```python
from build123d import *

# Parameters (mm, degrees)
SKETCH1_R           = 11.5
SKETCH1_R_2         = 1.75
BOSS_EXTRUDE1_DEPTH = 2
CUT_EXTRUDE1_DEPTH  = 2
CHAMFER1_SIZE       = 4
CHAMFER1_SIZE2      = 1.865230633
CHAMFER2_SIZE       = 4
CHAMFER2_SIZE2      = 1.865230633


with BuildPart() as part:
    # Sketch1 → Boss-Extrude1 (new body)
    with BuildSketch(Plane(origin=(0, 0, 0), x_dir=(1, 0, 0), z_dir=(0, 1, 0))):
        with Locations(Location((0, 0, 0), (0, 0, 270))):
            Circle(SKETCH1_R)
        with Locations(Location((0, 0, 0), (0, 0, 270))):
            Circle(SKETCH1_R_2, mode=Mode.SUBTRACT)
    extrude(amount=BOSS_EXTRUDE1_DEPTH)

    # Sketch2 → Cut-Extrude1 (cut)
    with BuildSketch(Plane(origin=(0, 2, 0), x_dir=(1, 0, 0), z_dir=(0, 1, 0))):
        with BuildLine():
            Line((-1.45362124, 4.5746022), (-2.346992627, 7.386076469))
            ThreePointArc((-2.346992627, 7.386076469), (-4.178678051, 6.526955626), (-5.725593472, 5.223033543))
            Line((-5.725593472, 5.223033543), (-3.546174021, 3.234911098))
            ThreePointArc((-3.546174021, 3.234911098), (-2.58808447, 4.042501549), (-1.45362124, 4.5746022))
        make_face()
        with BuildLine():
            Line((5.725593472, -5.223033543), (3.546174021, -3.234911098))
            ThreePointArc((3.546174021, -3.234911098), (2.58808447, -4.042501549), (1.45362124, -4.5746022))
            Line((1.45362124, -4.5746022), (2.346992627, -7.386076469))
            ThreePointArc((2.346992627, -7.386076469), (4.178678051, -6.526955626), (5.725593472, -5.223033543))
        make_face()
    extrude(amount=-CUT_EXTRUDE1_DEPTH, mode=Mode.SUBTRACT)

    # Chamfer1
    chamfer1_edges = [part.edges().sort_by_distance(p)[0] for p in [
        (-1.900306933, 2, -5.980339335),
    ]]
    chamfer1_side = [part.faces().sort_by_distance(p)[0] for p in [
        (0, 2, -11.174730881),
    ]]
    chamfer(chamfer1_edges, length=CHAMFER1_SIZE, length2=CHAMFER1_SIZE2, reference=chamfer1_side[0])

    # Chamfer2
    chamfer2_edges = [part.edges().sort_by_distance(p)[0] for p in [
        (1.900306933, 2, 5.980339335),
    ]]
    chamfer2_side = [part.faces().sort_by_distance(p)[0] for p in [
        (-0.343824977, 2, -4.461502083),
    ]]
    chamfer(chamfer2_edges, length=CHAMFER2_SIZE, length2=CHAMFER2_SIZE2, reference=chamfer2_side[0])


solid = part.part
```
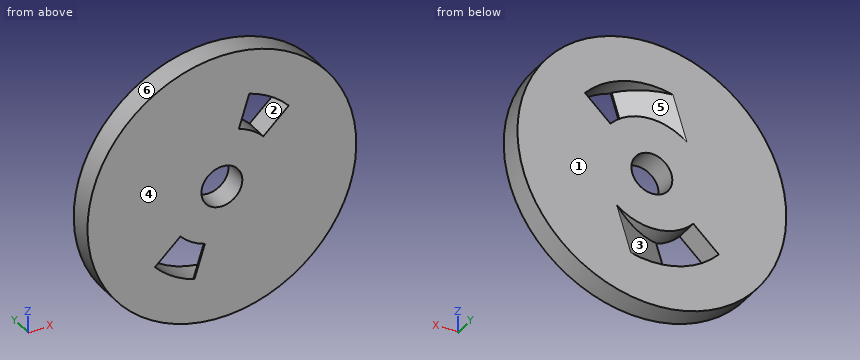
Can you work these out from the model? Positions are in its coordinate system, mm. Face numbers are marked on the shaded views. A direction names the side the tool comes from. Coordinates: 2 decimals unless noted, no trailing zeros. Loops run counter-clockwise (first coordinate to the right, second up) from the corner with the lowest first, then second, coordinate; pieces in that order, holes last. Notation, with made-up numbers: (25, 81.25) -> (81, 81.25) arc R33 ccw to (81, 110.25) -> close; hole circle Ø5 at (16.25, 71.5). An arc over 180 degrees is marked (long way). Answer as a JSON object with one key per item and string values.
1) If I drill on line 1 (Z direction, x = -3.75, y = 1.1); line 2 (X direction, y = 1.1, z = 3.5); line 3 (X direction, y = 0.5, z = 0), over which ranges is the centre line in solid material (lowest first)?
Results:
{"line 1": "z = -10.87 to -6.78, -3.42 to 10.87", "line 2": "x = -10.95 to 3.28, 3.84 to 10.95", "line 3": "x = -11.5 to -1.75, 1.75 to 11.5"}
2) For P1, Ø3, axis at x = 0, z = 0, coming from the -Y side, with a flat end and sliding along its axis, tell me the tip position at first contact or that it passes through.
Results:
{"P1": "passes through"}
3) Imagine slicing it at D-D (x = -5). Please give me the cut outline in (y, z), then the cut area to 3 significant figures.
Results:
{"outline": "(0, -10.36) -> (2, -10.36) -> (2, -5.92) -> (0, -5.92) -> close; (0, -4.56) -> (2, -4.56) -> (2, 10.36) -> (0, 10.36) -> close", "area": "38.7 mm^2"}
4) Imagine slicing it at B-B (x = 0). Please give me the cut outline in (y, z).
Results:
{"outline": "(0, -11.5) -> (2, -11.5) -> (2, -7.75) -> (1.23, -7.75) -> (0.81, -4.8) -> (2, -4.8) -> (2, -1.75) -> (0, -1.75) -> close; (0, 1.75) -> (2, 1.75) -> (2, 4.8) -> (0.81, 4.8) -> (1.23, 7.75) -> (2, 7.75) -> (2, 11.5) -> (0, 11.5) -> close"}
5) Imagine slicing it at C-C (y = 0.55). Please give me the cut outline in (x, z).
Results:
{"outline": "circle Ø23 at (0, 0); hole (-5.73, -5.22) arc R7.75 ccw to (-1.48, -7.61) -> (-0.58, -4.76) arc R4.8 cw to (-3.55, -3.23) -> close; hole circle Ø3.5 at (0, 0); hole (0.58, 4.76) arc R4.8 cw to (3.55, 3.23) -> (5.73, 5.22) arc R7.75 ccw to (1.48, 7.61) -> close"}
6) Thinking about a two-plate mould opening in Z: for the marked faces 4, 5 and 6, which applies, pulls with the +Z half, pulls with the -Z half, needs draft (parallel to the pull), parting line crosses it, or undercut?
Results:
{"face 4": "needs draft", "face 5": "undercut", "face 6": "parting line crosses it"}
7) For the marked faces 1, 2 and 3, which set-ups out of +Z, -Z, +X, -X, +Y, -Y let a thin tool reach every point of the face, with its end or its side?
Results:
{"face 1": "+Z, -Z, +X, -X, +Y", "face 2": "+Y, -Y", "face 3": "+Y"}
8) Imagine slicing it at A-A (z = 0). Please give me the cut outline in (x, y).
Results:
{"outline": "(-11.5, 0) -> (-1.75, 0) -> (-1.75, 2) -> (-11.5, 2) -> close; (1.75, 0) -> (11.5, 0) -> (11.5, 2) -> (1.75, 2) -> close"}
